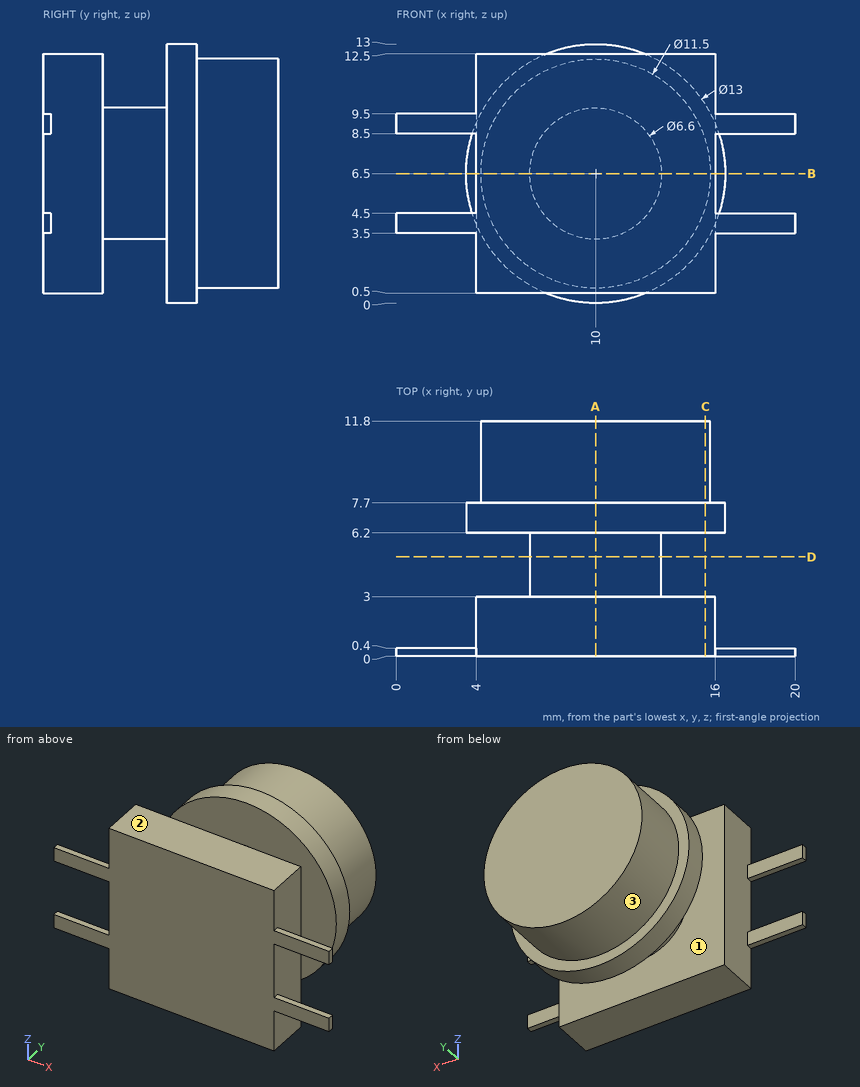
Could you check a few things on this drawing? It's one solid part, dimensions in mm from its lowest x, y, z. A direction names the side the tool comes from. Coordinates: 2 decimals unless noted, no trailing zeros. Write each loop counter-clockwise with the first axis right and the second up, starting at its lowest first coordinate (ties: lowest second). Pieces come first, ordered by that corner, then holes. Notation, with made-up numbers: M -33,-16 L 18,-16 A6 cw 18,-12 Z; hole C 10.5,-16 d6. An arc over 180 degrees is marked long. Answer as CSV lines item,"result". Start each with the question number.
Q1. Suppose I cut it at A-A, the plane x = 10. List the corners of the cut face in (y, z) for me, then the cut area to 3 significant figures.
Q2. Will these pins go through, and if not, where does the flat tip stop? pin 1 Ø5 at (x, y) = (9.5, 2.5) entering from +Z; pin 2 Ø5 at (y, z) = (6.5, 8) entering from +X; pin 3 Ø0.9 at (x, y) = (8.5, 1) entering from -Z.
Q3. Suppose I cut it at D-D, the plane y = 5. List the corners of the cut face in (x, z) for me.
Q4. Suppose I cut it at C-C, the plane x = 15.5. List the corners of the cut face in (y, z) for me.
Q5. For the marked faces 1, 2 and 3, which set-ups out of +Z, -Z, +X, -X, +Y, -Y let a thin tool reach every point of the face, with its end or its side?
Q6. Suppose I cut it at B-B, the plane z = 6.5. List the corners of the cut face in (x, y) for me.
Q7. I need wall thicknesses on probe 1 along Y at (x, z) = (14.75, 7.25); probe 2 along X at (y, z) = (1.5, 4); probe 3 along Y at (x, z) = (5.5, 1). Which ranges of each line are inside material? Lowest first, please. Write a range as [from, to].
Entries:
1,outline,"M 0,0.5 L 3,0.5 L 3,3.2 L 6.2,3.2 L 6.2,0 L 7.7,0 L 7.7,0.75 L 11.8,0.75 L 11.8,12.25 L 7.7,12.25 L 7.7,13 L 6.2,13 L 6.2,9.8 L 3,9.8 L 3,12.5 L 0,12.5 Z"
1,area,"124 mm²"
2,pin 1,"stops at z = 12.5"
2,pin 2,"stops at x = 16.5"
2,pin 3,"stops at z = 0.5"
3,outline,"C 10,6.5 d6.6"
4,outline,"M 0,0.5 L 3,0.5 L 3,12.5 L 0,12.5 Z; M 6.2,3.04 L 7.7,3.04 L 7.7,4.82 L 11.8,4.82 L 11.8,8.18 L 7.7,8.18 L 7.7,9.96 L 6.2,9.96 Z"
5,face 1,"none"
5,face 2,"+Z, +X, -X, -Y"
5,face 3,"+Y"
6,outline,"M 3.5,6.2 L 6.7,6.2 L 6.7,3 L 4,3 L 4,0 L 16,0 L 16,3 L 13.3,3 L 13.3,6.2 L 16.5,6.2 L 16.5,7.7 L 15.75,7.7 L 15.75,11.8 L 4.25,11.8 L 4.25,7.7 L 3.5,7.7 Z"
7,probe 1,"y = [0, 3], [6.2, 11.8]"
7,probe 2,"x = [4, 16]"
7,probe 3,"y = [0, 3]"
